from build123d import *

# Parameters (mm, degrees)
EXTRUDE1_DEPTH      = 13.7
EXTRUDE1_DEPTH_BACK = 13.7
SKETCH4_R           = 7.9375
EXTRUDE3_DEPTH      = 13.7
EXTRUDE3_DEPTH_BACK = 13.7
SKETCH5_R           = 9.525
EXTRUDE4_DEPTH      = 16.875
SKETCH6_R           = 4.7625
EXTRUDE5_DEPTH      = 88.9


with BuildPart() as part:
    # Sketch1 → Revolve1 (revolve)
    with BuildSketch(Plane.XY):
        with BuildLine():
            Line((-9.525, -9.516529567), (-9.525, -25.4254))
            ThreePointArc((-9.525, -25.4254), (-10.447496482, -27.652503518), (-12.6746, -28.575))
            Line((-12.6746, -28.575), (-12.7, -28.575))
            Line((-12.7, -28.575), (-12.7, -32.54375))
            ThreePointArc((-12.7, -32.54375), (-11.90625, -33.3375), (-12.7, -34.13125))
            Line((-12.7, -34.13125), (-12.7, -36.5125))
            Line((-12.7, -36.5125), (0, -36.5125))
            Line((0, -36.5125), (0, 12.7))
            ThreePointArc((0, 12.7), (-11.360741372, 5.676579559), (-10.155929487, -7.625424333))
            ThreePointArc((-10.155929487, -7.625424333), (-9.68689312, -8.519740845), (-9.525, -9.516529567))
        make_face()
    revolve(axis=Axis((0, 29.568581121, 0), (0, -1, 0)))

    # Sketch2 → Extrude1 (cut, two sides)
    with BuildSketch(Plane.XY) as extrude1_sk:
        Polygon((-6.35, 10.998522628), (-6.35, -11.1125), (-9.525, -22.225), (-17.461272298, -22.225), (-17.461272298, 15.422387348), (17.461272298, 15.422387348), (17.461272298, -22.225), (9.525, -22.225), (6.35, -11.1125), (6.35, 10.998522628), (6.35, 13.9933427), (-6.35, 13.9933427), align=None)
    extrude(amount=EXTRUDE1_DEPTH, mode=Mode.SUBTRACT)
    extrude(extrude1_sk.sketch, amount=-EXTRUDE1_DEPTH_BACK, mode=Mode.SUBTRACT)

    # Sketch4 → Extrude3 (cut, two sides)
    with BuildSketch(Plane(origin=(0, 0, 0), x_dir=(0, 0, -1), z_dir=(1, 0, 0))) as extrude3_sk:
        Circle(SKETCH4_R)
    extrude(amount=EXTRUDE3_DEPTH, mode=Mode.SUBTRACT)
    extrude(extrude3_sk.sketch, amount=-EXTRUDE3_DEPTH_BACK, mode=Mode.SUBTRACT)

    # Sketch5 → Extrude4 (cut, through all)
    with BuildSketch(Plane.ZY.offset(3.175)):
        Circle(SKETCH5_R)
    extrude(amount=-EXTRUDE4_DEPTH, mode=Mode.SUBTRACT)

    # Sketch6 → Extrude5 (add)
    with BuildSketch(Plane.XZ.offset(36.5125)):
        Circle(SKETCH6_R)
    extrude(amount=EXTRUDE5_DEPTH)


solid = part.part
Can you work these out from the model? Positions are in its coordinate system, mm. A direction names the side the tool comes from. Give positions to 0.01 mm unless a question says otherwise; leave off trailing zeros. Order: outer loops, then holes, each group sorted by start corner. A loop starts at its lowest first (then second) coordinate and runs counter-clockwise, first axis right, second up. Notation, with made-up numbers: M 87,77.5 L 91,77.5 A23 ccw 91,103.5 Z; hole C 43,-16.5 d6. An arc over 180 degrees is marked long. One line per question, with ' | ' between items.
Item 1: Suppose I cut it at D-D, the plane y = -68.5. Write out the boundary of the cut face in (x, z) (1 decimal), then the cut area to 3 significant figures.
Answer block:
outline: C 0,0 d9.5 | area: 71.3 mm2
Item 2: Please list where these lines run through material, in increasing order: L1, parallel to Y at x = 2.5, z = 0 (1 decimal); L2, parallel to Y at x = -4.15, z = 0; L3, parallel to Y at x = -11, z = 4.
Answer block:
L1: y = -125.4 to -9.5, 9.5 to 12.5 | L2: y = -125.41 to -7.94, 7.94 to 12 | L3: y = -36.51 to -28.42
Item 3: I'm going to push flat-ended pins straight in: pin 1 Ø5 at (y, z) = (-42.5, 4) entering from -X; pin 2 Ø12 at (x, z) = (-3, 4) entering from -Y; pin 3 Ø1.5 at (x, y) = (-4, -14) entering from +Z; pin 4 Ø4 at (x, z) = (-8, 7.5) entering from -Y. Where does each tip first touch, or does it pass through?
Answer block:
pin 1: stops at x = -4.52 | pin 2: stops at y = -125.41 | pin 3: stops at z = 8.95 | pin 4: stops at y = -36.51
Item 4: We'd pull the mould along Y, two halves only. Please class faces 4 (the face through (1.521, -5.796, -7.559)), 5 (the face through (-7.562, -15.356, -0.099)), 6 (the face through (-3.175, 8, -2)), 7 (the face through (-6.35, -8, -3)): released by +Y, released by -Y, zero draft, split by the parting line, or undercut.
Answer block:
face 4: undercut | face 5: released by +Y | face 6: undercut | face 7: zero draft
Item 5: For faces 1 (the face through (6.35, -10, 1)), 2 (the face through (7.02, -19.35, -6.44)), 3 (the face through (-5, -36.513, 0)), which set-ups out of +Z, -Z, +X, -X, +Y, -Y let a thin tool reach every point of the face, with its end or its side?
Answer block:
face 1: +Z, -Z, +X, +Y | face 2: none | face 3: -Y
